```python
from build123d import *

# Parameters (mm, degrees)
SKETCH2_R          = 1.25
CUT_EXTRUDE1_DEPTH = 5


with BuildPart() as part:
    # Sketch1 → Revolve1 (revolve)
    with BuildSketch(Plane(origin=(0, 0, 0), x_dir=(1, 0, 0), z_dir=(0, 1, 0))):
        Polygon((8.936305636, 8.625), (8.936305636, 14.031614125), (4.936305636, 15.92728698), (4.936305636, 16.55), (-11.063694364, 16.55), (-11.063694364, 18.55), (-12.563694364, 18.55), (-12.563694364, 16.55), (-12.563694364, 14.55), (3.172405145, 14.55), (7.050606918, 12.712049543), (7.050606918, 7.1), (8.936305636, 7.1), align=None)
    revolve(axis=Axis((-37.278866169, 0, 0), (1, 0, 0)))

    # Sketch2 → Cut-Extrude1 (cut)
    with BuildSketch(Plane(origin=(8.936305636, 0, 0), x_dir=(0, 0, -1), z_dir=(1, 0, 0))):
        with Locations((0, 10)):
            Circle(SKETCH2_R)
        with Locations((7.071067812, 7.071067812)):
            Circle(SKETCH2_R)
        with Locations((10, 0)):
            Circle(SKETCH2_R)
        with Locations((7.071067812, -7.071067812)):
            Circle(SKETCH2_R)
        with Locations((0, -10)):
            Circle(SKETCH2_R)
        with Locations((-7.071067812, -7.071067812)):
            Circle(SKETCH2_R)
        with Locations((-10, 0)):
            Circle(SKETCH2_R)
        with Locations((-7.071067812, 7.071067812)):
            Circle(SKETCH2_R)
    extrude(amount=-CUT_EXTRUDE1_DEPTH, mode=Mode.SUBTRACT)


solid = part.part
```
The listing builds one solid part. Answer for the finished solid, in the listing's coordinates (mm). A direction names the side the tool comes from. Give positions to 0.01 mm unless a question says otherwise; leave off trailing zeros. Order: outer loops, then holes, each group sorted by start corner. A loop starts at its lowest first (then second) coordinate and runs counter-clockwise, first axis right, second up. Notation, with made-up numbers: (28, 80.25) - (37, 80.25) arc R20 ccw to (37, 108.25) - close; hole circle Ø10 at (0, -15). An arc over 180 degrees is marked (long way). Use one line per item in the form item = value. Start each with the question number.
(1) The mould has two halves that part along Y. Classify faces 4 (the cylindrical face through (-4.585, 14.426, 1.894)), 5 (the cylindrical face through (-11.824, 18.392, 2.415)), 6 (the flat face through (-11.064, 0, -17)), 7 (the cylindrical face through (8.007, -6.226, 7.992)): released by +Y, released by -Y, zero draft, split by the parting line, or undercut.
(2) For faces 1 (the cylindrical face through (-3.176, -16.156, 3.588)), 2 (the flat face through (7.051, -5.5, -5.5)), 3 (the cylindrical face through (8.007, -8.946, -0.672)), determine the directions among +Z, -Z, +X, -X, +Y, -Y from which every point of the face is accessible in a straight line to the end or side of a thin tool.
(3) A cutting plane is placed at A-A, the plane y = 0. State how many separate pieces and enclosed holes the cut face has, then the cut area to 3 significant figures.
(4) Flat-ended cylindrical pins translate along their axes: pin 1 Ø6 at (y, z) = (-14, -3) entering from -X; pin 2 Ø4 at (y, z) = (-7.07, 7.07) entering from -X; pin 3 Ø1.5 at (x, z) = (0.5, 10) entering from +Y; pin 4 Ø1 at (x, y) = (-8, -13.5) entering from +Z. Find the tip coordinate at first contact, or state that the pin passes through.
(5) A cutting plane is placed at C-C, the plane x = 1.25. Write down the section's boundary in (y, z).
(6) Consider line 1 (Y direction, x = 7.8, z = 0); line 2 (Z direction, x = 7.75, y = 6.5); line 3 (Y direction, x = -5.5, z = 0). Determine where each line is inside the solid, lowest interval first. Write a range as from..to.
Ans:
q1.face_4 = undercut
q1.face_5 = split by the parting line
q1.face_6 = zero draft
q1.face_7 = undercut
q2.face_1 = +X
q2.face_2 = -X
q2.face_3 = +X, -X
q3.separate_pieces = 4
q3.enclosed_holes = 0
q3.area = 105 mm^2
q4.pin_1 = -12.56
q4.pin_2 = 7.05
q4.pin_3 = 13.72
q4.pin_4 = 10.24
q5.outline = circle Ø33.1 at (0, 0); hole circle Ø29.1 at (0, 0)
q6.line_1 = -14.57..-11.25, -8.75..-7.1, 7.1..8.75, 11.25..14.57
q6.line_2 = -13.07..-8.18, -5.96..-2.86, 2.86..5.96, 8.18..13.07
q6.line_3 = -16.55..-14.55, 14.55..16.55
